Verification items for the finished model (mm, model axes). Round coordinates to 2 decimals unless told otherwise and drop trailing zeros. Loops run counter-clockwise (first coordinate to the right, second up) from the corner with the lowest first, then second, coordinate; pieces in that order, holes last. Notation, with made-up numbers: M 45.5,36 L 64.5,36 A33 ccw 64.5,66 Z; hole C 66.5,1 d9. An arc over 180 degrees is marked long. One line per item, written item: value.
from build123d import *

# Parameters (mm, degrees)
SKETCH2_R           = 49.784
BOSS_EXTRUDE1_DEPTH = 203.2
SKETCH3_R           = 11.74839717
BOSS_EXTRUDE2_DEPTH = 50.8
SKETCH4_R           = 53.885165976
CUT_EXTRUDE1_DEPTH  = 375.969043164
SHELL1_T            = -3.175


with BuildPart() as part:
    # Sketch1 → Revolve1 (revolve)
    with BuildSketch(Plane.XY):
        with BuildLine():
            Line((304.8, 49.784), (304.8, 0))
            Line((304.8, 0), (0, 0))
            Line((0, 0), (0, 11.748397173))
            add(Edge.make_bspline(
                [(0, 11.748397173), (0.424160675, 11.855932678), (1.277768006, 12.07173392), (3.085410505, 12.527272667), (5.106222596, 13.032281093), (7.110128552, 13.529344024), (9.159948224, 14.034387922), (11.195444228, 14.532141119), (13.233412884, 15.026861964), (15.805049223, 15.64653599), (18.91026091, 16.387291474), (22.550652523, 17.244690048), (26.727238439, 18.213147263), (31.952168035, 19.405675489), (42.412897925, 21.742539102), (62.333903875, 25.976370199), (110.770450737, 35.225121195), (160.70732909, 42.159920913), (207.702302928, 46.434962608), (245.168015054, 48.368183749), (253.734807707, 48.740972714), (260.161369668, 48.98354131), (264.446272339, 49.130442523), (268.731666265, 49.262530797), (273.017475857, 49.379804553), (277.303691578, 49.48226239), (281.590188304, 49.569903083), (285.329649653, 49.633426545), (288.521672796, 49.67849525), (291.166731437, 49.70980578), (293.263778354, 49.731088433), (295.359186858, 49.74882407), (297.470177021, 49.76301264), (299.535126271, 49.773654103), (301.617177871, 49.780748429), (303.482211221, 49.783408805), (304.362420109, 49.784), (304.8, 49.784)],
                knots=[0.082917815, 0.082917815, 0.082917815, 0.082917815, 0.082917815, 0.088601511, 0.094285207, 0.099968902, 0.105652598, 0.111336294, 0.11701999, 0.122703686, 0.128387381, 0.140005218, 0.151623054, 0.16324089, 0.174858727, 0.198094396, 0.267801409, 0.383979763, 0.709279153, 0.744132659, 0.778986165, 0.790604, 0.802221836, 0.813839671, 0.825457507, 0.837075342, 0.848693177, 0.860311013, 0.871928848, 0.877612544, 0.883296239, 0.888979935, 0.89466363, 0.900347326, 0.906031021, 0.911714717, 0.917398412, 0.917398412, 0.917398412, 0.917398412, 0.917398412], degree=4))
        make_face()
    revolve(axis=Axis((304.8, 0, 0), (-1, 0, 0)))

    # Sketch2 → Boss-Extrude1 (add)
    with BuildSketch(Plane(origin=(304.8, 0, 0), x_dir=(0, 0, -1), z_dir=(1, 0, 0))):
        with Locations(Location((0, 0, 0), (0, 0, 90))):
            Circle(SKETCH2_R)
    extrude(amount=BOSS_EXTRUDE1_DEPTH)

    # Sketch3 → Boss-Extrude2 (add)
    with BuildSketch(Plane.ZY):
        with Locations(Location((0, 0, 0), (0, 0, 270))):
            Circle(SKETCH3_R)
    extrude(amount=BOSS_EXTRUDE2_DEPTH)

    # Sketch4 → Cut-Extrude1 (cut, through all)
    with BuildSketch(Plane(origin=(317.5, 0, 0), x_dir=(0, 0, -1), z_dir=(1, 0, 0))):
        Circle(SKETCH4_R)
    extrude(amount=-CUT_EXTRUDE1_DEPTH, mode=Mode.SUBTRACT)

    # Shell1
    shell1_openings = [part.faces().sort_by_distance(p)[0] for p in [
        (508, 0, 0),
        (317.5, 0, 0),
    ]]
    offset(amount=SHELL1_T, openings=shell1_openings, kind=Kind.INTERSECTION)


solid = part.part
(1) Thickness scan on L1, parallel to Z at x = 368, y = 0; L2, parallel to Y at x = 432, z = -29. Record the ranges inside material, lowest first. Write a range as from..to.
Completed:
L1: z = -49.78..-46.61, 46.61..49.78
L2: y = -40.47..-36.49, 36.49..40.47
(2) Depth check by flat-ended pin: pin 1 Ø2 at (x, y) = (355.5, 30.5) entering from -Z; pin 2 Ø10 at (x, z) = (352.5, 27.5) entering from +Y; pin 3 Ø6 at (x, y) = (407, 19.5) entering from -Z. Enter the tip coordinate at first touch or a pass-through.
Completed:
pin 1: stops at z = -40.1
pin 2: stops at y = 44.41
pin 3: stops at z = -46.97
(3) Sectioned sample at A-A on z = 0. Enter the section's corners in (x, y).
Completed:
outline: M 317.5,-49.78 L 508,-49.78 L 508,-46.61 L 317.5,-46.61 Z; M 317.5,46.61 L 508,46.61 L 508,49.78 L 317.5,49.78 Z
(4) Sectioned sample at C-C on x = 492.5. Enter the section's corners in (y, z), and give its area (3 significant figures).
Completed:
outline: C 0,0 d99.57; hole C 0,0 d93.22
area: 961 mm^2
(5) Mould release check, pull along Y, two halves, no side actions. Record for faces 1 (the face through (411.4, -10.8, -48.6)), 2 (the face through (411.416, -34.353, 31.501)), 3 (the face through (317.5, 44.5, -14.5)): +Y half, -Y half, draft (parallel to the pull), parting line (faces both ways), or undercut.
Completed:
face 1: parting line
face 2: undercut
face 3: draft
